from build123d import *

# Parameters (mm, degrees)
EXTRUDE_1_DEPTH     = 4
EXTRUDE_2_DEPTH     = 12
CUT_EXTRUDE_1_DEPTH = 6
CUT_EXTRUDE_START   = -20
CUT_EXTRUDE_2_DEPTH = 14
SKETCH_1_5_R        = 2.5
EXTRUDE_3_DEPTH     = 5
SKETCH_7_W          = 6
SKETCH_7_H          = 8
CUT_EXTRUDE_3_DEPTH = 25
FILLET_2_R          = 2


# Read off the part's stored shape, not the designer's step: 切除-拉伸2, 镜向1
with BuildPart() as part:
    # 草图1 → 凸台-拉伸1 (new body)
    with BuildSketch(Plane.XY):
        Polygon((-6.44865866, 2.619047619), (-6.44865866, 27.619047619), (-13.94865866, 27.619047619), (-13.94865866, 17.619047619), (-28.94865866, 17.619047619), (-28.94865866, -42.380952381), (-18.94865866, -42.380952381), (-18.94865866, -32.380952381), (-23.94865866, -32.380952381), (-23.94865866, 2.619047619), align=None)
    extrude(amount=EXTRUDE_1_DEPTH)

    # 草图1<4> → 凸台-拉伸2 (add)
    with BuildSketch(Plane.XY):
        Polygon((-13.94865866, 2.619047619), (-6.44865866, 2.619047619), (-6.44865866, 27.619047619), (-13.94865866, 27.619047619), (-13.94865866, 17.619047619), (-28.94865866, 17.619047619), (-28.94865866, -42.380952381), (-18.94865866, -42.380952381), (-18.94865866, -32.380952381), (-23.94865866, -32.380952381), (-23.94865866, 2.619047619), (-23.94865866, 12.619047619), (-13.94865866, 12.619047619), align=None)
    extrude(amount=-EXTRUDE_2_DEPTH)

    # 草图5 → 切除-拉伸1 (cut)
    with BuildSketch(Plane.XZ.offset(42.380952381)):
        with BuildLine():
            Line((-18.94865866, 4), (-23.425219682, 4))
            Line((-23.425219682, 4), (-24.77896144, 4))
            ThreePointArc((-24.77896144, 4), (-26.44865866, -4), (-24.77896144, -12))
            Line((-24.77896144, -12), (-18.94865866, -12))
            Line((-18.94865866, -12), (-18.94865866, 4))
        make_face()
    extrude(amount=-CUT_EXTRUDE_1_DEPTH, mode=Mode.SUBTRACT)

    # 切除-拉伸2 outline → 切除-拉伸2 (cut)
    with BuildSketch(Plane.XZ.offset(42.380952381).offset(CUT_EXTRUDE_START)):
        with BuildLine():
            ThreePointArc((-23.94865866, -1.4), (-25.493875387, -1.908994198), (-26.434087232, -3.236688257))
            ThreePointArc((-26.434087232, -3.236688257), (-26.44865866, -4), (-26.434087231, -4.763311743))
            ThreePointArc((-26.434087231, -4.763311743), (-25.493875387, -6.091005802), (-23.94865866, -6.6))
            Line((-23.94865866, -6.6), (-23.938488984, -8.05))
            Line((-23.938488984, -8.05), (-18.94865866, -8.05))
            Line((-18.94865866, -8.05), (-18.94865866, 0.05))
            Line((-18.94865866, 0.05), (-23.938488984, 0.05))
            Line((-23.938488984, 0.05), (-23.94865866, -1.4))
        make_face()
    extrude(amount=CUT_EXTRUDE_2_DEPTH, mode=Mode.SUBTRACT)

    # 草图1<5> → 凸台-拉伸3 (add)
    with BuildSketch(Plane.XY):
        with Locations((-18.94865866, 7.619047619)):
            Circle(SKETCH_1_5_R)
    extrude(amount=-EXTRUDE_3_DEPTH)

    # 镜向1: part across plane


with BuildPart() as part_1:
    add(part.part)
    add(part.part.mirror(Plane(origin=(-6.44865866, 0, 4), x_dir=(0, 0, 1), z_dir=(1, 0, 0))))

    # 草图7 → 切除-拉伸3 (cut)
    with BuildSketch(Plane(origin=(0, 27.619047619, 0), x_dir=(1, 0, 0), z_dir=(0, 1, 0))):
        with Locations((-6.44865866, 4)):
            Rectangle(SKETCH_7_W, SKETCH_7_H)
    extrude(amount=-CUT_EXTRUDE_3_DEPTH, mode=Mode.SUBTRACT)

    # 圆角2
    fillet_2_edges = [part_1.edges().sort_by_distance(p)[0] for p in [
        (16.05134134, -12.380952381, 4),
        (8.55134134, 17.619047619, 4),
        (16.05134134, 17.619047619, -4),
        (1.05134134, 22.619047619, 4),
        (1.05134134, 17.619047619, -4),
        (1.05134134, 22.619047619, -12),
        (8.55134134, 17.619047619, -12),
        (16.05134134, -12.380952381, -12),
        (-28.94865866, 17.619047619, -4),
        (-13.94865866, 17.619047619, -4),
        (-13.94865866, 22.619047619, 4),
        (-21.44865866, 17.619047619, 4),
        (-28.94865866, -12.380952381, 4),
        (-13.94865866, 22.619047619, -12),
        (-28.94865866, -12.380952381, -12),
        (-21.44865866, 17.619047619, -12),
    ]]
    fillet(fillet_2_edges, radius=FILLET_2_R)


solid = part_1.part
Check sheet for the modelled part. Datum: model origin and axes. Units: mm. A direction names the side the tool comes from. Coordinates: 2 decimals unless noted, no trailing zeros. Write each loop counter-clockwise with the first axis right and the second up, starting at its lowest first coordinate (ties: lowest second). Pieces come first, ordered by that corner, then holes.
Item 1: Mould release check, pull along X, two halves, no side actions. Record for faces 1 (the face through (8.63, 17.02, -11.43)), 2 (the face through (-28.347, -13.787, 3.43)), 3 (the face through (-18.949, -34, -10)): released by +X, released by -X, zero draft, split by the parting line, or undercut.
Numbers:
face 1: zero draft
face 2: released by -X
face 3: undercut
Item 2: Access from +Z, -Z, +X, -X, +Y, -Y to the whole of each face (thin tool, end or side, straight path). Record for faces 4 (the face through (10, -36.381, -9)), 5 (the face through (-19, 8, -5)), 6 (the face through (-13.949, 24, -4)).
Numbers:
face 4: -Y
face 5: -Z, -Y
face 6: +Z, -Z, -X, +Y
Item 3: Cross-section at C-C on x = -8.5. Record the boundary of the cut face in (y, z).
Numbers:
outline: (2.62, -12) - (27.62, -12) - (27.62, -8) - (2.62, -8) - close; (2.62, 0) - (27.62, 0) - (27.62, 4) - (2.62, 4) - close
Item 4: Scan lines: probe 1 along X at (y, z) = (11, -3.5); probe 2 along X at (y, z) = (-4, -7.5); probe 3 along Z at (x, y) = (-4, 9.5). Record each from-to range of solid material in increasing order.
Numbers:
probe 1: x = -28.95 to -23.95, -13.95 to -9.45, -3.45 to 1.05, 11.05 to 16.05
probe 2: x = -28.95 to -23.95, 11.05 to 16.05
probe 3: z = -12 to -8, 0 to 4
Item 5: Cross-section at D-D on z = 1. Record the boundary of the cut face in (x, y), then the cut area to 3 significant figures.
Numbers:
outline: (-28.95, -42.38) - (-25.81, -42.38) - (-25.81, -36.38) - (-18.95, -36.38) - (-18.95, -32.38) - (-23.95, -32.38) - (-23.95, 2.62) - (11.05, 2.62) - (11.05, -32.38) - (6.05, -32.38) - (6.05, -36.38) - (12.92, -36.38) - (12.92, -42.38) - (16.05, -42.38) - (16.05, 15.62) arc R2 ccw to (14.05, 17.62) - (3.05, 17.62) arc R2 cw to (1.05, 19.62) - (1.05, 27.62) - (-13.95, 27.62) - (-13.95, 19.62) arc R2 cw to (-15.95, 17.62) - (-26.95, 17.62) arc R2 ccw to (-28.95, 15.62) - close
area: 1,290 mm2
Item 6: Cross-section at B-B on y = 14. Record the boundary of the cut face in (x, z).
Numbers:
outline: (-28.95, -10) arc R2 ccw to (-26.95, -12) - (14.05, -12) arc R2 ccw to (16.05, -10) - (16.05, 2) arc R2 ccw to (14.05, 4) - (-26.95, 4) arc R2 ccw to (-28.95, 2) - close; hole (-9.45, -8) - (-3.45, -8) - (-3.45, 0) - (-9.45, 0) - close
Item 7: Cross-section at A-A on y = -0.5. Record the boundary of the cut face in (x, z).
Numbers:
outline: (-28.95, -10) arc R2 ccw to (-26.95, -12) - (-23.95, -12) - (-23.95, 4) - (-26.95, 4) arc R2 ccw to (-28.95, 2) - close; (11.05, -12) - (14.05, -12) arc R2 ccw to (16.05, -10) - (16.05, 2) arc R2 ccw to (14.05, 4) - (11.05, 4) - close
Item 8: Depth check by flat-ended pin: pin 1 Ø2 at (x, z) = (-15.5, -1.5) entering from +Y; pin 2 Ø5.5 at (x, y) = (5.5, 7.5) entering from -Z; pin 3 Ø2 at (x, y) = (-16, 17) entering from -Z. Enter the tip coordinate at first touch or a pass-through.
Numbers:
pin 1: stops at y = 18.24
pin 2: stops at z = -5
pin 3: stops at z = -11.96
